CAD build for the part. Positions are in the model's coordinates, mm. Face numbers are marked on the shaded views. A direction names the side the tool comes from. Round coordinates to 2 decimals unless told otherwise and drop trailing zeros. Loops run counter-clockwise (first coordinate to the right, second up) from the corner with the lowest first, then second, coordinate; pieces in that order, holes last.
```python
from build123d import *

# Parameters (mm, degrees)
SKETCH1_W           = 160
SKETCH1_H           = 120
BOSS_EXTRUDE1_DEPTH = 3
SKETCH2_W           = 160
SKETCH2_H           = 120
SKETCH2_W_2         = 156
SKETCH2_H_2         = 116
BOSS_EXTRUDE2_DEPTH = 50
SKETCH3_R           = 5
CUT_EXTRUDE1_DEPTH  = 179.910592196


with BuildPart() as part:
    # Sketch1 → Boss-Extrude1 (new body)
    with BuildSketch(Plane(origin=(0, 0, 0), x_dir=(1, 0, 0), z_dir=(0, 1, 0))):
        Rectangle(SKETCH1_W, SKETCH1_H)
    extrude(amount=BOSS_EXTRUDE1_DEPTH)

    # Sketch2 → Boss-Extrude2 (add)
    with BuildSketch(Plane(origin=(0, 3, 0), x_dir=(1, 0, 0), z_dir=(0, 1, 0))):
        Rectangle(SKETCH2_W, SKETCH2_H)
        Rectangle(SKETCH2_W_2, SKETCH2_H_2, mode=Mode.SUBTRACT)
    extrude(amount=BOSS_EXTRUDE2_DEPTH)

    # Sketch3 → Cut-Extrude1 (cut, through all)
    with BuildSketch(Plane(origin=(80, 0, 0), x_dir=(0, 0, -1), z_dir=(1, 0, 0))):
        with Locations((-26.5, 31.5)):
            Circle(SKETCH3_R)
    extrude(amount=-CUT_EXTRUDE1_DEPTH, mode=Mode.SUBTRACT)


solid = part.part
```
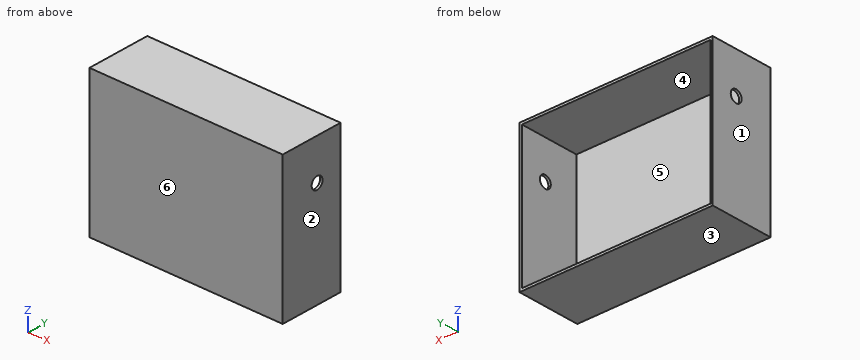
Item 1: Cut at C-C, the plane y = 41. Give the cut face in (x, z), plus the area to 3 significant figures.
Answers follow:
outline: (-80, -60) - (80, -60) - (80, 60) - (-80, 60) - close; hole (-78, -58) - (78, -58) - (78, 58) - (-78, 58) - close
area: 1,100 mm2
Item 2: Cut at A-A, the plane z = 26.5. Give the cut face in (x, y).
Answers follow:
outline: (-80, 0) - (80, 0) - (80, 26.5) - (78, 26.5) - (78, 3) - (-78, 3) - (-78, 26.5) - (-80, 26.5) - close; (-80, 36.5) - (-78, 36.5) - (-78, 53) - (-80, 53) - close; (78, 36.5) - (80, 36.5) - (80, 53) - (78, 53) - close
Item 3: 3-axis set-ups, long thin cutter, end or side, ignore diameter. For the marked faces 5 and 6: which of +Z, -Z, +X, -X, +Y, -Y reach the whole face in a straight line?
Answers follow:
face 5: +Y
face 6: +Z, -Z, +X, -X, -Y
Item 4: Probe line 1 (Z direction, x = -39.5, y = 49); line 2 (X direction, y = 18, z = 48); line 3 (Z direction, x = -79, y = 31). List the from-to ranges inside material, lowest first.
Answers follow:
line 1: z = -60 to -58, 58 to 60
line 2: x = -80 to -78, 78 to 80
line 3: z = -60 to 21.53, 31.47 to 60
Item 5: Cut at B-B, the plane y = 31.5. Give the cut face in (x, z), plus the area to 3 significant figures.
Answers follow:
outline: (-80, -60) - (80, -60) - (80, 21.5) - (78, 21.5) - (78, -58) - (-78, -58) - (-78, 21.5) - (-80, 21.5) - close; (-80, 31.5) - (-78, 31.5) - (-78, 58) - (78, 58) - (78, 31.5) - (80, 31.5) - (80, 60) - (-80, 60) - close
area: 1,060 mm2
Item 6: Two-plate mould, pull along X, no slides. Class the marked faces 1, 2, 3 and 4: released by +X, released by -X, zero draft, split by the parting line, or undercut.
Answers follow:
face 1: released by -X
face 2: released by +X
face 3: zero draft
face 4: undercut
Item 7: Cut at D-D, the plane z = -32.5. Give the cut face in (x, y), plus the area to 3 significant figures.
Answers follow:
outline: (-80, 0) - (80, 0) - (80, 53) - (78, 53) - (78, 3) - (-78, 3) - (-78, 53) - (-80, 53) - close
area: 680 mm2
